from build123d import *

# Parameters (mm, degrees)
EXTRUDE_1_DEPTH                  = 10
FILLET_1_R                       = 2
PATTERN_CIRCULAR_2_COUNT         = 3
FILLET_1_OF_PATTERN_CIRCULAR_2_R = 2
CUT_EXTRUDE_START                = -15
SKETCH_3_R                       = 51
CUT_EXTRUDE_1_DEPTH              = 15
SKETCH_4_R                       = 62.618720145
SKETCH_4_R_2                     = 57
CUT_EXTRUDE_2_DEPTH              = 15
CHAMFER_1_SIZE                   = 2
FILLET_2_R                       = 5
SKETCH_5_R                       = 42.5
EXTRUDE_2_DEPTH                  = 3
SKETCH_7_R                       = 39.5
CUT_EXTRUDE_3_DEPTH              = 3
EXTRUDE_START                    = 3
SKETCH_8_W                       = 3
SKETCH_8_H                       = 3
EXTRUDE_4_DEPTH                  = 3
SKETCH_9_R                       = 73.179522897
CUT_EXTRUDE_4_DEPTH              = 130


with BuildPart() as part:
    # Эскиз1 → Повернуть1 (revolve)
    with BuildSketch(Plane(origin=(0, 0, 0), x_dir=(1, 0, 0), z_dir=(0, 1, 0))):
        Polygon((0, 0), (-54, 0), (-54, 145), (-51, 145), (-51, 3), (0, 3), align=None)
    revolve(axis=Axis((0, 0, -3), (0, 0, 1)))

    # Эскиз2 → Бобышка-Вытянуть1 (add)
    with BuildSketch(Plane(origin=(57, 0, 0), x_dir=(0, 0, -1), z_dir=(1, 0, 0))):
        Polygon((145, 14), (145, -14), (140, -14), (138.5, 11), (134, 11), (134, 14), align=None)
    extrude_1 = extrude(amount=-EXTRUDE_1_DEPTH)

    # Скругление1
    fillet_1_edges = [part.edges().sort_by_distance(p)[0] for p in [
        (54.576809621, -14, -140),
    ]]
    fillet(fillet_1_edges, radius=FILLET_1_R)

    # Круговой массив2: Бобышка-Вытянуть1 ×3 about axis
    pattern_circular_2_axis = Axis((0, 0, 0), (0, 0, 1))
    for i in range(1, PATTERN_CIRCULAR_2_COUNT):
        add(extrude_1.rotate(pattern_circular_2_axis, i * 360 / PATTERN_CIRCULAR_2_COUNT))

    # Скругление1 of Круговой массив2
    fillet_1_of_pattern_circular_2_edges = [part.edges().sort_by_distance(p)[0] for p in [
        (-15.164049157, 54.264903589, -140),
        (-39.412760463, -40.264903589, -140),
    ]]
    fillet(fillet_1_of_pattern_circular_2_edges, radius=FILLET_1_OF_PATTERN_CIRCULAR_2_R)

    # Эскиз3 → Вырез-Вытянуть1 (cut)
    with BuildSketch(Plane(origin=(0, 0, -145), x_dir=(-1, 0, 0), z_dir=(0, 0, -1)).offset(CUT_EXTRUDE_START)):
        Circle(SKETCH_3_R)
    extrude(amount=CUT_EXTRUDE_1_DEPTH, mode=Mode.SUBTRACT)

    # Эскиз4 → Вырез-Вытянуть2 (cut)
    with BuildSketch(Plane(origin=(0, 0, -145), x_dir=(-1, 0, 0), z_dir=(0, 0, -1))):
        Circle(SKETCH_4_R)
        Circle(SKETCH_4_R_2, mode=Mode.SUBTRACT)
    extrude(amount=-CUT_EXTRUDE_2_DEPTH, mode=Mode.SUBTRACT)

    # Фаска1
    chamfer_1_edges = [part.edges().sort_by_distance(p)[0] for p in [
        (54, 0, 0),
    ]]
    chamfer(chamfer_1_edges, length=CHAMFER_1_SIZE)

    # Скругление2
    fillet_2_edges = [part.edges().sort_by_distance(p)[0] for p in [
        (51, 0, -3),
    ]]
    fillet(fillet_2_edges, radius=FILLET_2_R)

    # Эскиз5 → Бобышка-Вытянуть2 (add)
    with BuildSketch(Plane.XY):
        Circle(SKETCH_5_R)
    extrude(amount=EXTRUDE_2_DEPTH)

    # Эскиз7 → Вырез-Вытянуть3 (cut)
    with BuildSketch(Plane.XY.offset(3)):
        Circle(SKETCH_7_R)
    extrude(amount=-CUT_EXTRUDE_3_DEPTH, mode=Mode.SUBTRACT)

    # Эскиз8 → Бобышка-Вытянуть4 (add)
    with BuildSketch(Plane.XY.offset(EXTRUDE_START)):
        with BuildLine():
            Line((-1.5, -7.858116823), (-1.5, -39.471508712))
            ThreePointArc((-1.5, -39.471508712), (0, -39.5), (1.5, -39.471508712))
            Line((1.5, -39.471508712), (1.5, -7.858116823))
            ThreePointArc((1.5, -7.858116823), (0, -8), (-1.5, -7.858116823))
        make_face()
        with BuildLine():
            ThreePointArc((1.5, 39.471508712), (0, 39.5), (-1.5, 39.471508712))
            Line((-1.5, 39.471508712), (-1.5, 7.858116823))
            ThreePointArc((-1.5, 7.858116823), (0, 8), (1.5, 7.858116823))
            Line((1.5, 7.858116823), (1.5, 39.471508712))
        make_face()
        with BuildLine():
            Line((-1.5, 7.858116823), (-1.5, 1.5))
            Line((-1.5, 1.5), (1.5, 1.5))
            Line((1.5, 1.5), (1.5, 7.858116823))
            ThreePointArc((1.5, 7.858116823), (0, 8), (-1.5, 7.858116823))
        make_face()
        with BuildLine():
            Line((1.5, 7.858116823), (1.5, 1.5))
            Line((1.5, 1.5), (7.858116823, 1.5))
            ThreePointArc((7.858116823, 1.5), (5.656854249, 5.656854249), (1.5, 7.858116823))
        make_face()
        with BuildLine():
            Line((1.5, 1.5), (1.5, -1.5))
            Line((1.5, -1.5), (7.858116823, -1.5))
            ThreePointArc((7.858116823, -1.5), (7.964450219, -0.753347668), (8, 0))
            ThreePointArc((8, 0), (7.964450219, 0.753347668), (7.858116823, 1.5))
            Line((7.858116823, 1.5), (1.5, 1.5))
        make_face()
        with BuildLine():
            ThreePointArc((-39.471508712, 1.5), (-39.5, 0), (-39.471508712, -1.5))
            Line((-39.471508712, -1.5), (-7.858116823, -1.5))
            ThreePointArc((-7.858116823, -1.5), (-8, 0), (-7.858116823, 1.5))
            Line((-7.858116823, 1.5), (-39.471508712, 1.5))
        make_face()
        with BuildLine():
            Line((7.858116823, -1.5), (39.471508712, -1.5))
            ThreePointArc((39.471508712, -1.5), (39.492876536, -0.75013528), (39.5, 0))
            ThreePointArc((39.5, 0), (39.492876536, 0.75013528), (39.471508712, 1.5))
            Line((39.471508712, 1.5), (7.858116823, 1.5))
            ThreePointArc((7.858116823, 1.5), (7.964450219, 0.753347668), (8, 0))
            ThreePointArc((8, 0), (7.964450219, -0.753347668), (7.858116823, -1.5))
        make_face()
        with BuildLine():
            Line((1.5, -1.5), (1.5, -7.858116823))
            ThreePointArc((1.5, -7.858116823), (5.656854249, -5.656854249), (7.858116823, -1.5))
            Line((7.858116823, -1.5), (1.5, -1.5))
        make_face()
        with BuildLine():
            Line((-1.5, -1.5), (-1.5, -7.858116823))
            ThreePointArc((-1.5, -7.858116823), (0, -8), (1.5, -7.858116823))
            Line((1.5, -7.858116823), (1.5, -1.5))
            Line((1.5, -1.5), (-1.5, -1.5))
        make_face()
        Rectangle(SKETCH_8_W, SKETCH_8_H)
        with BuildLine():
            Line((-7.858116823, 1.5), (-1.5, 1.5))
            Line((-1.5, 1.5), (-1.5, 7.858116823))
            ThreePointArc((-1.5, 7.858116823), (-5.656854249, 5.656854249), (-7.858116823, 1.5))
        make_face()
        with BuildLine():
            Line((-7.858116823, -1.5), (-1.5, -1.5))
            Line((-1.5, -1.5), (-1.5, 1.5))
            Line((-1.5, 1.5), (-7.858116823, 1.5))
            ThreePointArc((-7.858116823, 1.5), (-8, 0), (-7.858116823, -1.5))
        make_face()
        with BuildLine():
            ThreePointArc((-7.858116823, -1.5), (-5.656854249, -5.656854249), (-1.5, -7.858116823))
            Line((-1.5, -7.858116823), (-1.5, -1.5))
            Line((-1.5, -1.5), (-7.858116823, -1.5))
        make_face()
    extrude(amount=-EXTRUDE_4_DEPTH)

    # Эскиз9 → Вырез-Вытянуть4 (cut)
    with BuildSketch(Plane(origin=(0, 0, -145), x_dir=(-1, 0, 0), z_dir=(0, 0, -1))):
        Circle(SKETCH_9_R)
    extrude(amount=-CUT_EXTRUDE_4_DEPTH, mode=Mode.SUBTRACT)


solid = part.part
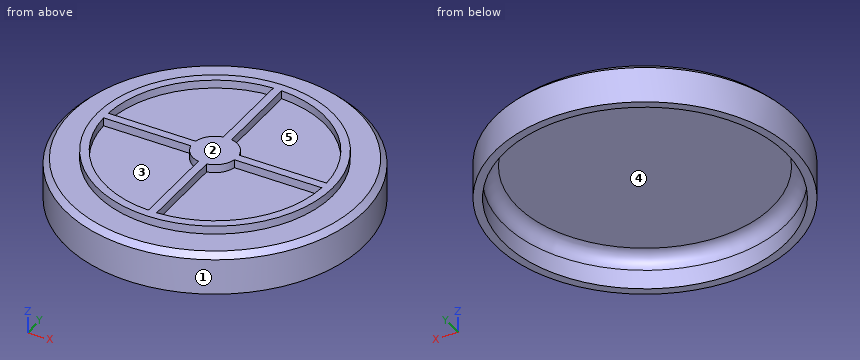
Here's how the part is built. I have some questions about the finished solid (model axes, mm). Face numbers are marked on the shaded views. A direction names the side the tool comes from. Round coordinates to 2 decimals unless told otherwise and drop trailing zeros. Order: outer loops, then holes, each group sorted by start corner. A loop starts at its lowest first (then second) coordinate and runs counter-clockwise, first axis right, second up. Notation, with made-up numbers: M 39,60.5 L 64,60.5 A14 cw 64,82.5 Z; hole C 77.5,29.25 d3. An arc over 180 degrees is marked long. One line per question, with ' | ' between items.
1) Imagine slicing it at D-D, the plane z = -5.75. Write out the boundary of the cut face in (x, y).
Checked values:
outline: C 0,0 d108; hole C 0,0 d100.93
2) I need wall thicknesses on line 1 (X direction, y = 0, z = -11.5); line 2 (X direction, y = -31, z = 1). Which ranges of each line are inside material? Lowest first, please.
Checked values:
line 1: x = -54 to -51, 51 to 54 | line 2: x = -29.07 to -24.48, -1.5 to 1.5, 24.48 to 29.07
3) We'd pull the mould along X, two halves only. Please class the marked faces 1, 2 and 3: released by +X, released by -X, zero draft, split by the parting line, or undercut.
Checked values:
face 1: split by the parting line | face 2: zero draft | face 3: undercut
4) I'm going to push flat-ended pins straight in: pin 1 Ø10 at (x, z) = (17, -7.5) entering from -Y; pin 2 Ø0.9 at (y, z) = (-18, 2) entering from +X; pin 3 Ø2.5 at (y, z) = (20.5, 1.5) entering from -X. Where does each tip first touch, or does it pass through?
Checked values:
pin 1: stops at y = -52.65 | pin 2: stops at x = 38.71 | pin 3: stops at x = -37.89
5) Imagine slicing it at C-C, the plane z = -13.5. Write out the boundary of the cut face in (x, y), plus the area to 3 significant figures.
Checked values:
outline: C 0,0 d108; hole C 0,0 d102 | area: 990 mm²
6) On a 3-axis mill with a long thin cutter (end or side, diameter ignored), from which of +Z, -Z, +X, -X, +Y, -Y can I reach the whole of each face in a straight line? I mean the marked faces 4 and 5. Say none if no direction works.
Checked values:
face 4: -Z | face 5: +Z
7) Imagine slicing it at A-A, the plane x = 0. Write out the boundary of the cut face in (y, z), plus the area to 3 significant figures.
Checked values:
outline: M -54,-15 L -51,-15 L -51,-8 A5 cw -46,-3 L 46,-3 A5 cw 51,-8 L 51,-15 L 54,-15 L 54,-2 L 52,0 L 42.5,0 L 42.5,3 L -42.5,3 L -42.5,0 L -52,0 L -54,-2 Z | area: 658 mm²
